from build123d import *

# Parameters (mm, degrees)
SKETCH_1_R               = 30
EXTRUDE_1_DEPTH          = 5
SKETCH_2_R               = 4.5
CUT_EXTRUDE_1_DEPTH      = 43.720018727
CUT_EXTRUDE_7_DEPTH      = 43.720018727
PATTERN_CIRCULAR_1_COUNT = 14
FILLET_3_R               = 2
SKETCH_4_R               = 22
CUT_EXTRUDE_9_DEPTH      = 0.1
CUT_EXTRUDE_START        = -0.1
SKETCH_5_R               = 22
CUT_EXTRUDE_10_DEPTH     = 0.1


with BuildPart() as part:
    # 草图1 → 凸台-拉伸1 (new body)
    with BuildSketch(Plane.XY):
        Circle(SKETCH_1_R)
    extrude(amount=EXTRUDE_1_DEPTH)

    # 草图2 → 切除-拉伸1 (cut, through all)
    with BuildSketch(Plane.XY.offset(5)):
        Circle(SKETCH_2_R)
    extrude(amount=-CUT_EXTRUDE_1_DEPTH, mode=Mode.SUBTRACT)

    # 草图3 → 切除-拉伸7 (cut, through all)
    with BuildSketch(Plane.XY):
        with BuildLine():
            Line((0, 23), (0, 30))
            ThreePointArc((0, 30), (-2.625482426, 29.884893208), (-5.230817461, 29.540456135))
            ThreePointArc((-5.230817461, 29.540456135), (-4.501731259, 27.437843644), (-3.656838203, 25.379032895))
            ThreePointArc((-3.656838203, 25.379032895), (-2.181299106, 23.647100626), (0, 23))
        make_face()
        with BuildLine():
            ThreePointArc((5.230817461, 29.540456135), (2.625482426, 29.884893208), (0, 30))
            Line((0, 30), (0, 23))
            ThreePointArc((0, 23), (2.181299106, 23.647100626), (3.656838203, 25.379032895))
            ThreePointArc((3.656838203, 25.379032895), (4.501731259, 27.437843644), (5.230817461, 29.540456135))
        make_face()
    cut_extrude_7 = extrude(amount=CUT_EXTRUDE_7_DEPTH, mode=Mode.SUBTRACT)

    # 阵列(圆周)1: 切除-拉伸7 ×14 about axis
    pattern_circular_1_axis = Axis((0, 0, 0), (0, 0, 1))
    for i in range(1, PATTERN_CIRCULAR_1_COUNT):
        add(cut_extrude_7.rotate(pattern_circular_1_axis, i * 360 / PATTERN_CIRCULAR_1_COUNT), mode=Mode.SUBTRACT)

    # 圆角3
    # the kernel refuses this fillet: 2 mm, written as the material it takes off along each edge
    with BuildSketch(Plane(origin=(5.230817461, 29.540456135, -4.577149267), x_dir=(-0.32171090906550515, -0.9468379433610834, 0), z_dir=(0, 0, 1)), Plane(origin=(-19.834297271, 22.507790913, -4.577149267), x_dir=(0.5396842419659282, -0.8418675186593562, 0), z_dir=(0, 0, 1)), Plane(origin=(-27.635848838, 11.673039835, -4.577149267), x_dir=(0.8515113273463623, -0.5243362083633328, 0), z_dir=(0, 0, 1)), Plane(origin=(-29.963781612, -1.473699943, -4.577149267), x_dir=(0.9946861512447445, -0.10295368143936073, 0), z_dir=(0, 0, 1)), Plane(origin=(-26.357019955, -14.328555373, -4.577149267), x_dir=(0.9408511838640222, 0.33882008473770825, 0), z_dir=(0, 0, 1)), Plane(origin=(-17.529927249, -24.345464683, -4.577149267), x_dir=(0.7006691007364907, 0.7134863777768412, 0), z_dir=(0, 0, 1)), Plane(origin=(-5.230817461, -29.540456135, -4.577149267), x_dir=(0.32171090906550703, 0.9468379433610828, 0), z_dir=(0, 0, 1)), Plane(origin=(8.104319877, -28.88459796, -4.577149267), x_dir=(-0.12096607367127866, 0.9926566420573404, 0), z_dir=(0, 0, 1)), Plane(origin=(19.834297271, -22.507790913, -4.577149267), x_dir=(-0.5396842419659312, 0.8418675186593543, 0), z_dir=(0, 0, 1)), Plane(origin=(27.635848838, -11.673039835, -4.577149267), x_dir=(-0.8515113273463634, 0.524336208363331, 0), z_dir=(0, 0, 1)), Plane(origin=(29.963781612, 1.473699943, -4.577149267), x_dir=(-0.9946861512447445, 0.10295368143936018, 0), z_dir=(0, 0, 1)), Plane(origin=(26.357019955, 14.328555373, -4.577149267), x_dir=(-0.9408511838640224, -0.3388200847377076, 0), z_dir=(0, 0, 1)), Plane(origin=(17.529927249, 24.345464683, -4.577149267), x_dir=(-0.7006691007364938, -0.7134863777768381, 0), z_dir=(0, 0, 1))) as fillet_3_piece_1:
        with BuildLine():
            CenterArc((1.769304863, 1.999534384), FILLET_3_R, 185.227747584, 83.53589182)
            ThreePointArc((-0.222375917, 1.817304657), (-0.125054645, 0.906955521), (0, 0))
            ThreePointArc((0, 0), (0.863075543, 0.009312326), (1.726151086, 0))
        make_face()
    extrude(amount=14.154298534, mode=Mode.SUBTRACT)
    with BuildSketch(Plane(origin=(-5.230817461, 29.540456135, -4.577149267), x_dir=(-0.9789028377703077, -0.20432629347501635, 0), z_dir=(0, 0, 1)), Plane(origin=(-17.529927249, 24.345464683, -4.577149267), x_dir=(-0.7933071253194062, -0.6088216527994549, 0), z_dir=(0, 0, 1)), Plane(origin=(-26.357019955, 14.328555373, -4.577149267), x_dir=(-0.4505872074255905, -0.8927324170793888, 0), z_dir=(0, 0, 1)), Plane(origin=(-29.963781612, 1.473699943, -4.577149267), x_dir=(-0.018622967011686854, -0.9998265775121612, 0), z_dir=(0, 0, 1)), Plane(origin=(-27.635848838, -11.673039835, -4.577149267), x_dir=(0.4170297804145827, -0.9088928222003764, 0), z_dir=(0, 0, 1)), Plane(origin=(-19.834297271, -22.507790913, -4.577149267), x_dir=(0.7700846652951304, -0.6379416966128542, 0), z_dir=(0, 0, 1)), Plane(origin=(-8.104319877, -28.88459796, -4.577149267), x_dir=(0.9706148377453508, -0.24063839416968846, 0), z_dir=(0, 0, 1)), Plane(origin=(5.230817461, -29.540456135, -4.577149267), x_dir=(0.9789028377703077, 0.20432629347501674, 0), z_dir=(0, 0, 1)), Plane(origin=(17.529927249, -24.345464683, -4.577149267), x_dir=(0.7933071253194082, 0.6088216527994523, 0), z_dir=(0, 0, 1)), Plane(origin=(26.357019955, -14.328555373, -4.577149267), x_dir=(0.45058720742559166, 0.8927324170793882, 0), z_dir=(0, 0, 1)), Plane(origin=(29.963781612, -1.473699943, -4.577149267), x_dir=(0.01862296701168685, 0.9998265775121612, 0), z_dir=(0, 0, 1)), Plane(origin=(27.635848838, 11.673039835, -4.577149267), x_dir=(-0.4170297804145869, 0.9088928222003745, 0), z_dir=(0, 0, 1)), Plane(origin=(19.834297271, 22.507790913, -4.577149267), x_dir=(-0.7700846652951312, 0.6379416966128533, 0), z_dir=(0, 0, 1)), Plane(origin=(8.104319877, 28.88459796, -4.577149267), x_dir=(-0.9706148377453518, 0.24063839416968458, 0), z_dir=(0, 0, 1))) as fillet_3_piece_2:
        with BuildLine():
            CenterArc((1.76983105, 1.999068659), FILLET_3_R, 188.212721849, 83.53589182)
            ThreePointArc((-0.209658025, 1.713371262), (-0.095585631, 0.857816705), (0, 0))
            ThreePointArc((0, 0), (0.915429853, -0.013970116), (1.830859707, 0))
        make_face()
    extrude(amount=14.154298534, mode=Mode.SUBTRACT)
    with BuildSketch(Plane(origin=(-8.104319877, 28.88459796, -4.577149267), x_dir=(0.9706148377453514, 0.24063839416968652, 0), z_dir=(0, 0, 1))) as fillet_3_piece_3:
        with BuildLine():
            CenterArc((1.76983105, -1.999068659), FILLET_3_R, 88.251386331, 83.53589182)
            ThreePointArc((-0.209658025, -1.713371262), (-0.095585631, -0.857816705), (0, 0))
            ThreePointArc((0, 0), (0.915429853, 0.013970116), (1.830859707, 0))
        make_face()
    extrude(amount=14.154298534, mode=Mode.SUBTRACT)

    # 草图4 → 切除-拉伸9 (cut)
    with BuildSketch(Plane.XY.offset(5)):
        Circle(SKETCH_4_R)
    extrude(amount=-CUT_EXTRUDE_9_DEPTH, mode=Mode.SUBTRACT)

    # 草图5 → 切除-拉伸10 (cut)
    with BuildSketch(Plane(origin=(0, 0, 0), x_dir=(-1, 0, 0), z_dir=(0, 0, -1)).offset(CUT_EXTRUDE_START)):
        with Locations(Location((0, 0, 0), (0, 0, 180))):
            Circle(SKETCH_5_R)
    extrude(amount=CUT_EXTRUDE_10_DEPTH, mode=Mode.SUBTRACT)


solid = part.part
For this review, take the finished solid that the model builds, in its own axes (mm). A direction names the side the tool comes from. Round coordinates to 2 decimals unless told otherwise and drop trailing zeros. Loops run counter-clockwise (first coordinate to the right, second up) from the corner with the lowest first, then second, coordinate; pieces in that order, holes last. Notation, with made-up numbers: (-15.5, 24.25) - (20.5, 24.25) arc R27 ccw to (20.5, 55.25) - close; hole circle Ø4 at (-7.5, -33.75). An arc over 180 degrees is marked (long way). Use one line per item in the form item = value.
Item 1: Consider section A-A on x = 11. Write out the cut boundary in (y, z), then the cut area to 3 significant figures.
Answers:
outline = (-20.39, 0) - (-19.05, 0) - (-19.05, 0.1) - (19.05, 0.1) - (19.05, 0) - (20.39, 0) - (20.39, 5) - (19.05, 5) - (19.05, 4.9) - (-19.05, 4.9) - (-19.05, 5) - (-20.39, 5) - close
area = 196 mm^2
Item 2: Mouldability with a two-part tool opening along X and no side actions: class faces 1 (the cylindrical face through (-26.879, -1.847, 2.465)), 2 (the cylindrical face through (7.612, -28.413, 2.465)), 3 (the cylindrical face through (-15.315, -22.166, 2.465)) as +X half, -X half, draft (parallel to the pull), parting line (faces both ways), or undercut.
Answers:
face_1 = -X half
face_2 = +X half
face_3 = undercut
Item 3: For line 1 (Y direction, x = -18, z = 2.2); line 2 (Y direction, x = 0, z = 2.5); line 3 (Y direction, x = 0, z = 4.95), list the stretches that pass through material, from the lowest coordinate up.
Answers:
line_1 = -23.66 to -19.5, -14.32 to 14.32, 19.5 to 23.66
line_2 = -23 to -4.5, 4.5 to 23
line_3 = -23 to -22, 22 to 23
Item 4: Tool access review of faces 4 (the cylindrical face through (-23.416, -13.326, 2.465)), 5 (the cylindrical face through (-26.92, 1.84, 2.46)), 6 (the cylindrical face through (7.78, -25.79, 2.46)): name each direction out of +Z, -Z, +X, -X, +Y, -Y from which nothing blocks a thin tool from reaching the whole face with its end or side.
Answers:
face_4 = +Z, -Z, -Y
face_5 = +Z, -Z, -X
face_6 = +Z, -Z, +X
Item 5: Clearance check with flat-ended pins moving along their axes: P1, Ø12, axis at x = -0.5, y = -4.5, coming from the +Z side; P2, Ø8, axis at x = 0, y = 0, coming from the +Z side; P3, Ø3, axis at y = -22, z = 3.5, coming from the -X side; P4, Ø13, axis at x = 10.5, y = 6.5, coming from the -Z side. State where each tip first meets the part, or that it passes through.
Answers:
P1 = 4.9
P2 = through
P3 = -19.2
P4 = 0.1
